Read the model definition and answer for the solid it produces. Units are mm, in the model's axes. Give positions to 0.01 mm unless a question says otherwise; leave off trailing zeros. Loops run counter-clockwise (first coordinate to the right, second up) from the corner with the lowest first, then second, coordinate; pieces in that order, holes last. Notation, with made-up numbers: (-25, 65) -> (-21, 65) arc R24 ccw to (-21, 89) -> close; hole circle Ø1 at (63.5, 36). An arc over 180 degrees is marked (long way). Return JSON: item names as keys, results as strings. Group by question number.
from build123d import *

# Parameters (mm, degrees)
SKETCH_R   = 1.5
SKETCH_R_2 = 3.25
PAD_DEPTH  = 1.6


with BuildPart() as part:
    # Sketch → Pad (new body)
    with BuildSketch(Plane.XY):
        with BuildLine():
            Line((20.5, 0), (20.5, 20))
            Line((20.5, 20), (0, 20))
            Line((0, 20), (0, -40))
            Line((0, -40), (-55, -40))
            Line((-55, -40), (-69.142136, -25.857864))
            Line((-69.142136, -25.857864), (-69.142136, 4.142136))
            Line((-69.142136, 4.142136), (-90, 25))
            Line((-90, 25), (-106.464466, 25))
            Line((-106.464466, 25), (-110, 28.535534))
            Line((-110, 28.535534), (-110, 56.464466))
            Line((-110, 56.464466), (-106.464466, 60))
            Line((-106.464466, 60), (-10, 60))
            Line((-10, 60), (0, 50))
            Line((0, 50), (40, 50))
            ThreePointArc((90, 0), (75.355339, 35.355339), (40, 50))
            Line((20.5, 0), (90, 0))
        make_face()
        with Locations((56, 6)):
            Circle(SKETCH_R, mode=Mode.SUBTRACT)
        with Locations((-8, 52)):
            Circle(SKETCH_R, mode=Mode.SUBTRACT)
        with Locations((-78, 40)):
            Circle(SKETCH_R, mode=Mode.SUBTRACT)
        with Locations((-4, 16)):
            Circle(SKETCH_R, mode=Mode.SUBTRACT)
        with Locations((-67, 10)):
            Circle(SKETCH_R, mode=Mode.SUBTRACT)
        with Locations((-30, 27)):
            Circle(SKETCH_R_2, mode=Mode.SUBTRACT)
        with Locations((-46, 5)):
            Circle(SKETCH_R, mode=Mode.SUBTRACT)
        with Locations((-14, 5)):
            Circle(SKETCH_R, mode=Mode.SUBTRACT)
        with Locations((-14, -5)):
            Circle(SKETCH_R, mode=Mode.SUBTRACT)
        with Locations((-46, -5)):
            Circle(SKETCH_R, mode=Mode.SUBTRACT)
    extrude(amount=PAD_DEPTH)


solid = part.part
1. Flat-ended cylindrical pins translate along their axes: pin 1 Ø2.5 at (x, y) = (-14, 5) entering from -Z; pin 2 Ø0.5 at (y, z) = (9, 0.5) entering from -X; pin 3 Ø0.8 at (x, z) = (60.5, 0.5) entering from -Y; pin 4 Ø0.8 at (x, z) = (-100, 0.5) entering from -Y. Find the tip coordinate at first contact, or state that the pin passes through.
2. Straight lines are drawn through the part: line 1 (Y direction, x = -14, z = 1.4); line 2 (Y direction, x = -30.5, z = 1.3); line 3 (Y direction, x = 28.5, z = 0.45). For each, find the intervals that lie inside material, in ascending order. Write a range as from..to.
3. Section A-A on z = 0.3 is taken. State how many separate pieces and enclosed holes the cut face has, then the cut area to 3 significant figures.
4. Section B-B on x = -72 is taken. Determine the outline of the cut face in (y, z), then the cut area to 3 significant figures.
5. Section C-C on y = -31.5 is taken. Determine the outline of the cut face in (x, z).
Completed:
{
 "1": {"pin 1": "passes through", "pin 2": "stops at x = -74.25", "pin 3": "stops at y = 0", "pin 4": "stops at y = 25"},
 "2": {"line 1": "y = -40..-6.5, -3.5..3.5, 6.5..60", "line 2": "y = -40..23.79, 30.21..60", "line 3": "y = 0..50"},
 "3": {"separate pieces": "1", "enclosed holes": "10", "area": "11,900 mm²"},
 "4": {"outline": "(7, 0) -> (60, 0) -> (60, 1.6) -> (7, 1.6) -> close", "area": "84.8 mm²"},
 "5": {"outline": "(-63.5, 0) -> (0, 0) -> (0, 1.6) -> (-63.5, 1.6) -> close"}
}
